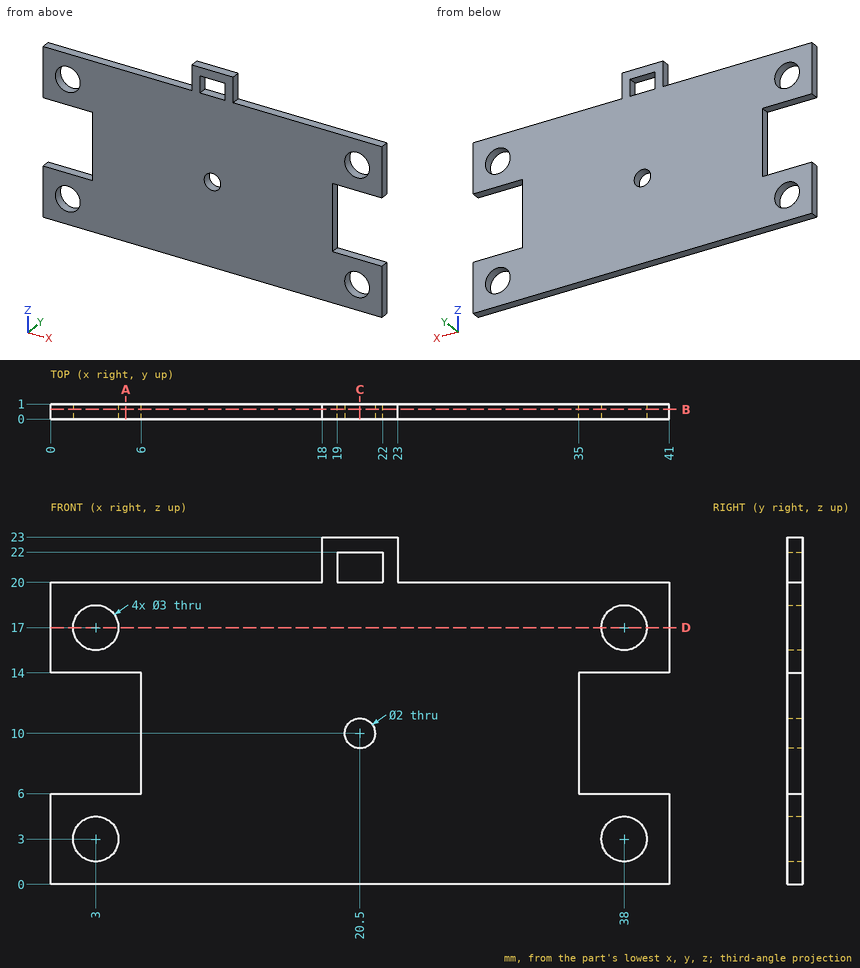
Geometry: see drawing. Coordinates: mm, zero at the bounding-box minimum. Coordinates: 2 decimals unless noted, no trailing zeros. Loops run counter-clockwise (first coordinate to the right, second up) from the corner with the lowest first, then second, coordinate; pieces in that order, holes last.
Q1. Contact query for flat-ended pins moving along their axis: pin 1 (0.5 mm diameter, centred on x = 1.5, y = 0.5, fed in from +Z); pin 2 (2.5 mm diameter, centred on x = 38, z = 3, fed in from +Y) (1 decimal); pin 3 (0.5 mm diameter, centred on y = 0.5, z = 9, fed in from -X). Output: stop coordinate, or through.
Q2. Cut plane C-C (x = 20.5). Output: boundary loops of the cut face in (y, z), then the cut area to 3 significant figures.
Q3. Cut plane D-D (z = 17). Output: boundary loops of the cut face in (x, y), then the cut area to 3 significant figures.
Q4. Cut plane B-B (y = 0.65). Output: boundary loops of the cut face in (x, z).
Q5. Material intervals for line 1 (X direction, y = 0.75, z = 17); line 2 (X direction, y = 0.5, z = 10); line 3 (X direction, y = 0.15, z = 20.25), sorted ascending.
Q6. Cut plane A-A (x = 5). Output: boundary loops of the cut face in (y, z).
Working result:
1. pin 1: stops at z = 20
1. pin 2: passes through
1. pin 3: stops at x = 6
2. outline: (0, 0) - (1, 0) - (1, 9) - (0, 9) - close; (0, 11) - (1, 11) - (1, 20) - (0, 20) - close; (0, 22) - (1, 22) - (1, 23) - (0, 23) - close
2. area: 19.0 mm2
3. outline: (0, 0) - (1.5, 0) - (1.5, 1) - (0, 1) - close; (4.5, 0) - (36.5, 0) - (36.5, 1) - (4.5, 1) - close; (39.5, 0) - (41, 0) - (41, 1) - (39.5, 1) - close
3. area: 35.0 mm2
4. outline: (0, 0) - (41, 0) - (41, 6) - (35, 6) - (35, 14) - (41, 14) - (41, 20) - (23, 20) - (23, 23) - (18, 23) - (18, 20) - (0, 20) - (0, 14) - (6, 14) - (6, 6) - (0, 6) - close; hole circle Ø3 at (3, 3); hole circle Ø3 at (3, 17); hole (19, 20) - (22, 20) - (22, 22) - (19, 22) - close; hole circle Ø2 at (20.5, 10); hole circle Ø3 at (38, 3); hole circle Ø3 at (38, 17)
5. line 1: x = 0 to 1.5, 4.5 to 36.5, 39.5 to 41
5. line 2: x = 6 to 19.5, 21.5 to 35
5. line 3: x = 18 to 19, 22 to 23
6. outline: (0, 0) - (1, 0) - (1, 6) - (0, 6) - close; (0, 14) - (1, 14) - (1, 20) - (0, 20) - close
